from build123d import *

# Parameters (mm, degrees)
VACIADO1_T              = -2
CROQUIS2_R              = 10
SALIENTE_EXTRUIR1_DEPTH = 2
CROQUIS3_R              = 10
SALIENTE_EXTRUIR2_DEPTH = 2
CROQUIS4_W              = 80.821615775
CROQUIS4_H              = 80
CORTAR_EXTRUIR1_DEPTH   = 50


with BuildPart() as part:
    # Croquis1 → Revolución1 (revolve)
    with BuildSketch(Plane.XY):
        with BuildLine():
            Line((0, 35), (10, 35))
            add(Edge.make_bspline(
                [(10, -35), (62.5, 0), (10, 35)],
                knots=[3.5531095, 3.5531095, 3.5531095, 5.871668461, 5.871668461, 5.871668461], degree=2, weights=[1, 0.4, 1]))
            Line((10, -35), (0, -35))
            Line((0, -35), (0, 0))
            Line((0, 0), (0, 35))
        make_face()
    revolve(axis=Axis((0, 0, 0), (0, 1, 0)))

    # Vaciado1
    vaciado1_openings = [part.faces().sort_by_distance(p)[0] for p in [
        (0, 35, 0),
        (0, -35, 0),
    ]]
    offset(amount=VACIADO1_T, openings=vaciado1_openings)

    # Croquis2 → Saliente-Extruir1 (add)
    with BuildSketch(Plane(origin=(0, 35, 0), x_dir=(1, 0, 0), z_dir=(0, 1, 0))):
        Circle(CROQUIS2_R)
    extrude(amount=-SALIENTE_EXTRUIR1_DEPTH)

    # Croquis3 → Saliente-Extruir2 (add)
    with BuildSketch(Plane.XZ.offset(35)):
        Circle(CROQUIS3_R)
    extrude(amount=-SALIENTE_EXTRUIR2_DEPTH)

    # Croquis4 → Cortar-Extruir1 (cut)
    with BuildSketch(Plane.XY):
        with Locations((2.983348233, -0.749824732)):
            Rectangle(CROQUIS4_W, CROQUIS4_H)
    extrude(amount=-CORTAR_EXTRUIR1_DEPTH, mode=Mode.SUBTRACT)


solid = part.part
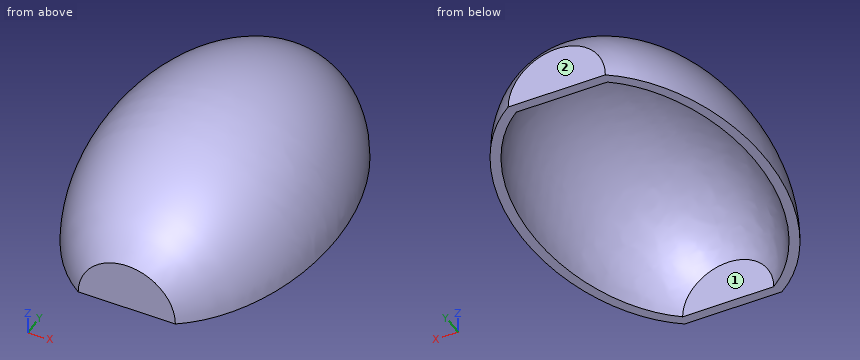
Read the model definition and answer for the solid it produces. Units are mm, in the model's axes. Face numbers are marked on the shaded views. Round coordinates to 2 decimals unless told otherwise and drop trailing zeros.
1. Straight lines are drawn through the part: L1, parallel to X at y = -1.5, z = 7.75; L2, parallel to Y at x = 11, z = 11.25; L3, parallel to Y at x = -19, z = 2.75. For each, find the intervals that lie inside material, in ascending order.
2. Given pin 1 Ø12 at (y, z) = (-2.5, 19) entering from +X; pin 2 Ø5 at (y, z) = (13, 15) entering from -X; pin 3 Ø12 at (y, z) = (-1.5, 17.5) entering from +X; pin 4 Ø1 at (y, z) = (-25.5, 20) entering from +X, each flat-ended and moving along its own axis, determine where each tip first touches the part or whether it passes through.
3. Determine the mould class of the marked faces 1 and 2 for opening direction X: pulls with the +X half, pulls with the -X half, needs draft (parallel to the pull), parting line crosses it, or undercut.
Values:
1. L1: x = -23.75 to -21.63, 21.63 to 23.75
1. L2: y = -29.68 to -26.31, 26.31 to 29.68
1. L3: y = -24.46 to -19.85, 19.85 to 24.46
2. pin 1: stops at x = 21.3
2. pin 2: stops at x = -20.04
2. pin 3: stops at x = 22.18
2. pin 4: passes through
3. face 1: undercut
3. face 2: needs draft
